Geometry check sheet. Reference: the model listing, model coordinates, mm. Face numbers are marked on the shaded views. A direction names the side the tool comes from. Round coordinates to 2 decimals unless told otherwise and drop trailing zeros. Write each loop counter-clockwise with the first axis right and the second up, starting at its lowest first coordinate (ties: lowest second). Pieces come first, ordered by that corner, then holes.
Item 1: Access from +Z, -Z, +X, -X, +Y, -Y to the whole of each face (thin tool, end or side, straight path). Record for the marked faces 4 and 5.
Item 2: Cross-section at A-A (y = 26.5). Enter the section's corners in (x, z) (1 decimal), then the cut area to 3 significant figures.
Item 3: Cross-section at C-C (x = -82.5). Enter the section's corners in (y, z) (3 decimals).
Item 4: Cross-section at B-B (z = -65.5). Enter the section's corners in (x, y) (3 decimals).
Item 5: Depth check by flat-ended pin: P1, Ø2.5, axis at x = -38.3, y = 51.5, coming from the +Z side; P2, Ø6, axis at x = -35, y = 73.5, coming from the +Z side; P3, Ø2.5, axis at x = -68.9, z = -42.95, coming from the +Y side (3 decimals). Enter the tip coordinate at first touch or a pass-through.
Item 6: Scan lines: probe 1 along Z at (x, y) = (-32.7, 95.5); probe 2 along X at (y, z) = (97, -109.45); probe 3 along Y at (x, z) = (-52.5, -54.5) (3 decimals). Record each from-to range of solid material in increasing order.
Item 7: Draft check along Y on the marked faces 1, 2 and 3. Enter one of: pulls with the +Y half, pulls with the -Y half, needs draft (parallel to the pull), parting line crosses it, or undercut.
Item 8: Cross-section at D-D (y = 44.5). Enter the section's corners in (x, z) (3 decimals), then the cut area to 3 significant figures.
Autodesk Inventor part; units mm, degrees
ref_plane "YZ Plane" through (0, 0, 0) normal (1, 0, 0) x (0, 1, 0)
ref_plane "XZ Plane" through (0, 0, 0) normal (0, 1, 0) x (-1, 0, 0)
ref_plane "XY Plane" through (0, 0, 0) normal (0, 0, 1) x (1, 0, 0)
sketch "Sketch1" plane through (0, 0, 0) normal (1, 0, 0) x (0, 1, 0)
  line L0 (6.35, 0) -> (95.25, 0)
  line L1 (101.6, -6.35) -> (101.6, -146.05)
  line L2 (95.25, -152.4) -> (6.35, -152.4)
  line L3 (0, -146.05) -> (0, -6.35)
  arc A0 (101.6, -6.35) -> (95.25, 0) centre (95.25, -6.35) ccw
  arc A1 (95.25, -152.4) -> (101.6, -146.05) centre (95.25, -146.05) ccw
  arc A2 (0, -146.05) -> (6.35, -152.4) centre (6.35, -146.05) ccw
  arc A3 (6.35, 0) -> (0, -6.35) centre (6.35, -6.35) ccw
  line L4 (92.075, -142.875) -> (92.075, -9.525)
  line L5 (92.075, -9.525) -> (9.525, -9.525)
  line L6 (9.525, -9.525) -> (9.525, -142.875)
  line L7 (9.525, -142.875) -> (92.075, -142.875)
  point P0 (0, 0)
  point P1 (101.6, -152.4)
  point P2 (101.6, 0)
  point P3 (0, -152.4)
  dimension "d0" = 101.6
  dimension "d1" = 152.4
  dimension "d2" = 6.35
  dimension "d3" = 6.35
  dimension "d4" = 9.525
extrude "Extrusion1" add sketch "Sketch1" against normal blind 101.6
sketch "Sketch2" plane through (0, 101.6, -6.35) normal (0, 1, 0) x (1, 0, 0)
  line L0 (0, 0) -> (0, 139.7) construction
  line L1 (0, 69.85) -> (-101.6, 69.85) construction
  line L2 (-101.6, 139.7) -> (-101.6, 0) construction
  line L3 (0, 99.6) -> (-45.4, 99.6) construction
  line L4 (-45.4, 99.6) -> (-45.4, 126.6) construction
  line L5 (-45.4, 126.6) -> (0, 126.6) construction
  line L6 (0, 126.6) -> (0, 99.6) construction
  line L7 (-32.7, 123.1) -> (-12.7, 123.1) construction
  line L8 (-12.7, 123.1) -> (-12.7, 103.1) construction
  line L9 (-12.7, 103.1) -> (-32.7, 103.1) construction
  line L10 (-32.7, 103.1) -> (-32.7, 123.1) construction
  line L11 (-32.7, 123.1) -> (-32.7, 126.6) construction
  line L12 (-32.7, 123.1) -> (-45.4, 123.1) construction
  line L13 (-12.7, 103.1) -> (-12.7, 99.6) construction
  line L14 (-12.7, 103.1) -> (0, 103.1) construction
  circle A0 centre (-32.7, 123.1) radius 1.6
  circle A1 centre (-12.7, 123.1) radius 1.6
  circle A2 centre (-12.7, 103.1) radius 1.6
  circle A3 centre (-32.7, 103.1) radius 1.6
  line L15 (0, 139.7) -> (0, 0) construction
  line L16 (-50.8, 69.85) -> (-50.8, 128.3257) construction
  line L17 (-101.6, 99.6) -> (-56.2, 99.6) construction
  line L18 (-56.2, 99.6) -> (-56.2, 126.6) construction
  line L19 (-56.2, 126.6) -> (-101.6, 126.6) construction
  line L20 (-101.6, 126.6) -> (-101.6, 99.6) construction
  line L21 (-68.9, 123.1) -> (-88.9, 123.1) construction
  line L22 (-88.9, 123.1) -> (-88.9, 103.1) construction
  line L23 (-88.9, 103.1) -> (-68.9, 103.1) construction
  line L24 (-68.9, 103.1) -> (-68.9, 123.1) construction
  line L25 (-68.9, 123.1) -> (-68.9, 126.6) construction
  line L26 (-68.9, 123.1) -> (-56.2, 123.1) construction
  line L27 (-88.9, 103.1) -> (-88.9, 99.6) construction
  line L28 (-88.9, 103.1) -> (-101.6, 103.1) construction
  circle A4 centre (-68.9, 123.1) radius 1.6
  circle A5 centre (-88.9, 123.1) radius 1.6
  circle A6 centre (-88.9, 103.1) radius 1.6
  circle A7 centre (-68.9, 103.1) radius 1.6
  line L29 (0, 40.1) -> (-45.4, 40.1) construction
  line L30 (-45.4, 40.1) -> (-45.4, 13.1) construction
  line L31 (-45.4, 13.1) -> (0, 13.1) construction
  line L32 (0, 13.1) -> (0, 40.1) construction
  line L33 (-32.7, 16.6) -> (-12.7, 16.6) construction
  line L34 (-12.7, 16.6) -> (-12.7, 36.6) construction
  line L35 (-12.7, 36.6) -> (-32.7, 36.6) construction
  line L36 (-32.7, 36.6) -> (-32.7, 16.6) construction
  line L37 (-32.7, 16.6) -> (-32.7, 13.1) construction
  line L38 (-32.7, 16.6) -> (-45.4, 16.6) construction
  line L39 (-12.7, 36.6) -> (-12.7, 40.1) construction
  line L40 (-12.7, 36.6) -> (0, 36.6) construction
  circle A8 centre (-32.7, 16.6) radius 1.6
  circle A9 centre (-12.7, 16.6) radius 1.6
  circle A10 centre (-12.7, 36.6) radius 1.6
  circle A11 centre (-32.7, 36.6) radius 1.6
  line L41 (-68.9, 16.6) -> (-88.9, 16.6) construction
  line L42 (-88.9, 36.6) -> (-68.9, 36.6) construction
  line L43 (-88.9, 36.6) -> (-88.9, 40.1) construction
  line L44 (-88.9, 16.6) -> (-88.9, 36.6) construction
  circle A12 centre (-88.9, 36.6) radius 1.6
  circle A13 centre (-88.9, 16.6) radius 1.6
  line L45 (-101.6, 40.1) -> (-56.2, 40.1) construction
  line L46 (-101.6, 13.1) -> (-101.6, 40.1) construction
  line L47 (-88.9, 36.6) -> (-101.6, 36.6) construction
  line L48 (-56.2, 13.1) -> (-101.6, 13.1) construction
  line L49 (-68.9, 36.6) -> (-68.9, 16.6) construction
  line L50 (-68.9, 16.6) -> (-68.9, 13.1) construction
  circle A14 centre (-68.9, 16.6) radius 1.6
  circle A15 centre (-68.9, 36.6) radius 1.6
  line L51 (-56.2, 40.1) -> (-56.2, 13.1) construction
  line L52 (-68.9, 16.6) -> (-56.2, 16.6) construction
  point P0 (0, -6.35)
  dimension "d7" = 45.4
  dimension "d8" = 27
  dimension "d9" = 20
  dimension "d10" = 20
  dimension "d11" = 3.2
  dimension "d12" = 3.2
  dimension "d13" = 3.2
  dimension "d14" = 3.2
  dimension "d15" = 106.5
extrude "Extrusion2" cut sketch "Sketch2" against normal up to next
sketch "Sketch3" plane through (0, 6.35, -152.4) normal (0, 0, -1) x (-1, 0, 0)
  line L0 (38.3, 45.15) -> (63.3, 45.15) construction
  line L1 (63.3, 45.15) -> (63.3, 20.15) construction
  line L2 (63.3, 20.15) -> (38.3, 20.15) construction
  line L3 (38.3, 20.15) -> (38.3, 45.15) construction
  circle A0 centre (38.3, 45.15) radius 2.1
  circle A1 centre (63.3, 45.15) radius 2.1
  circle A2 centre (63.3, 20.15) radius 2.1
  circle A3 centre (38.3, 20.15) radius 2.1
  line L4 (0, -6.35) -> (101.6, -6.35) construction
  line L5 (38.3, 32.65) -> (0, 32.65) construction
  line L6 (0, 0) -> (0, 88.9) construction
  line L7 (63.3, 32.65) -> (101.6, 32.65) construction
  line L8 (101.6, 88.9) -> (101.6, 0) construction
  dimension "d18" = 25
  dimension "d19" = 25
  dimension "d20" = 4.2
  dimension "d21" = 4.2
  dimension "d22" = 4.2
  dimension "d23" = 4.2
  dimension "d24" = 26.5
extrude "Extrusion3" cut sketch "Sketch3" against normal up to next
sketch "Sketch4" plane through (0, 6.35, 0) normal (0, 0, 1) x (1, 0, 0)
  line L0 (-88.9, 80.5892) -> (-12.7, 80.5892) construction
  line L1 (-12.7, 80.5892) -> (-12.7, 10.7392) construction
  line L2 (-12.7, 10.7392) -> (-88.9, 10.7392) construction
  line L3 (-88.9, 10.7392) -> (-88.9, 80.5892) construction
  line L4 (-88.9, 80.5892) -> (-88.9, 97.6783) construction
  line L5 (-88.9, 80.5892) -> (-101.6, 80.5892) construction
  line L6 (-101.6, 85.725) -> (-101.6, 3.175) construction
  line L7 (-12.7, 10.7392) -> (-12.7, -6.35) construction
  line L8 (0, -6.35) -> (-101.6, -6.35) construction
  line L9 (-12.7, 10.7392) -> (0, 10.7392) construction
  line L10 (0, 85.725) -> (0, 3.175) construction
  circle A0 centre (-12.7, 80.5892) radius 3.175
  circle A1 centre (-12.7, 10.7392) radius 3.175
  circle A2 centre (-88.9, 10.7392) radius 3.175
  circle A3 centre (-88.9, 80.5892) radius 3.175
  circle A4 centre (-63.3, 45.15) radius 2.1
  circle A5 centre (-63.3, 20.15) radius 2.1
  circle A6 centre (-38.3, 45.15) radius 2.1
  circle A7 centre (-38.3, 20.15) radius 2.1
  circle A8 centre (-63.3, 45.15) radius 4.7625
  circle A9 centre (-38.3, 45.15) radius 2.1
  circle A10 centre (-38.3, 45.15) radius 4.7625
  circle A11 centre (-63.3, 20.15) radius 2.1
  circle A12 centre (-63.3, 20.15) radius 4.7625
  circle A13 centre (-38.3, 20.15) radius 2.1
  circle A14 centre (-38.3, 20.15) radius 4.7625
  dimension "d27" = 6.35
  dimension "d28" = 6.35
  dimension "d29" = 6.35
  dimension "d30" = 6.35
  dimension "d31" = 69.85
  dimension "d32" = 76.2
  dimension "d33" = 9.525
  dimension "d34" = 9.525
  dimension "d35" = 9.525
  dimension "d36" = 9.525
extrude "Extrusion4" cut sketch "Sketch4" against normal up to next contours A0 | A1 | A2 | A3 | A4 | A5 | A6 | A7 | A8 | A10 | A12 | A14
thread "Thread1"
thread "Thread2"
thread "Thread3"
thread "Thread4"
sketch "Sketch5" plane through (0, 101.6, -6.35) normal (0, 1, 0) x (1, 0, 0)
  line L0 (21.1594, 98.325) -> (-128.3175, 98.325) construction
  line L1 (0, 146.05) -> (-101.6, 146.05) construction
  circle A0 centre (-32.7, 103.1) radius 1.6 construction
  circle A1 centre (-32.7, 103.1) radius 2.75 construction
  line L2 (0, 3.175) -> (0, 136.525) construction
  line L3 (-101.6, 136.525) -> (-101.6, 3.175) construction
  line L4 (0, 98.325) -> (-101.6, 98.325) construction
  line L5 (-101.6, 98.325) -> (-101.6, 73.325) construction
  line L6 (-101.6, 73.325) -> (0, 73.325) construction
  line L7 (0, 73.325) -> (0, 98.325) construction
  line L8 (-43.3, 78.325) -> (-58.3, 78.325) construction
  line L9 (-58.3, 78.325) -> (-58.3, 93.325) construction
  line L10 (-58.3, 93.325) -> (-43.3, 93.325) construction
  line L11 (-43.3, 93.325) -> (-43.3, 78.325) construction
  line L12 (-43.3, 78.325) -> (0, 78.325) construction
  line L13 (-58.3, 93.325) -> (-101.6, 93.325) construction
  line L14 (-58.3, 93.325) -> (-58.3, 98.325) construction
  line L15 (-43.3, 78.325) -> (-43.3, 73.325) construction
  circle A2 centre (-43.3, 78.325) radius 3.175
  circle A3 centre (-58.3, 78.325) radius 3.175
  circle A4 centre (-58.3, 93.325) radius 3.175
  circle A5 centre (-43.3, 93.325) radius 3.175
  point P0 (0, -6.35)
  dimension "d47" = 47.725
  dimension "d48" = 5.5
  dimension "d49" = 25
  dimension "d50" = 15
  dimension "d51" = 15
  dimension "d52" = 6.35
  dimension "d53" = 6.35
  dimension "d54" = 6.35
  dimension "d55" = 6.35
extrude "Extrusion5" cut sketch "Sketch5" against normal up to next
thread "Thread5"
thread "Thread6"
thread "Thread7"
thread "Thread8"
equation "\"d12\" = d11"
equation "\"d13\" = d11"
equation "\"d14\" = d11"
equation "\"d16\" = d12"
equation "\"d21\" = d20"
equation "\"d22\" = d20"
equation "\"d23\" = d20"
equation "\"d34\" = d33"
equation "\"d35\" = d33"
equation "\"d36\" = d33"
equation "\"d37\" = d33"
equation "\"d53\" = d52"
equation "\"d54\" = d52"
equation "\"d55\" = d52"
properties part number "4in x 6in Steel Rectangular Tubing 4in long Machined"
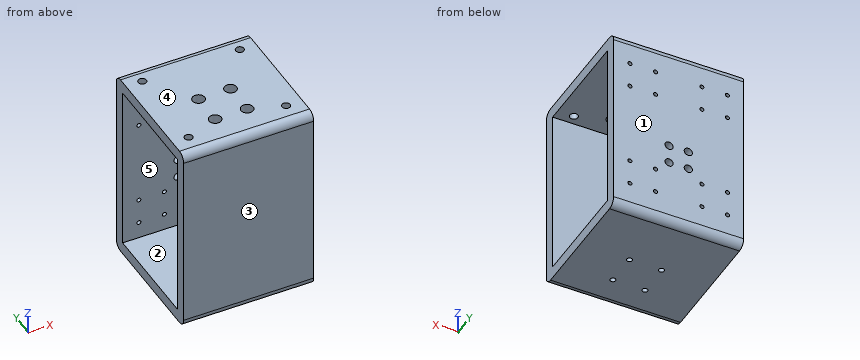
Resolved:
1. face 4: +Z, +X, -X, +Y, -Y
1. face 5: +X, -X
2. outline: (-101.6, -152.4) - (-65.4, -152.4) - (-65.4, -142.9) - (-101.6, -142.9) - close; (-101.6, -9.5) - (-68.1, -9.5) - (-68.1, 0) - (-101.6, 0) - close; (-61.2, -152.4) - (-40.4, -152.4) - (-40.4, -142.9) - (-61.2, -142.9) - close; (-58.5, -9.5) - (-43.1, -9.5) - (-43.1, 0) - (-58.5, 0) - close; (-36.2, -152.4) - (0, -152.4) - (0, -142.9) - (-36.2, -142.9) - close; (-33.5, -9.5) - (0, -9.5) - (0, 0) - (-33.5, 0) - close
2. area: 1,670 mm2
3. outline: (0, -146.05) arc R6.35 ccw to (6.35, -152.4) - (95.25, -152.4) arc R6.35 ccw to (101.6, -146.05) - (101.6, -6.35) arc R6.35 ccw to (95.25, 0) - (6.35, 0) arc R6.35 ccw to (0, -6.35) - close; hole (9.525, -142.875) - (92.075, -142.875) - (92.075, -9.525) - (9.525, -9.525) - close
4. outline: (-101.6, 0) - (0, 0) - (0, 9.525) - (-101.6, 9.525) - close; (-101.6, 92.075) - (0, 92.075) - (0, 101.6) - (-101.6, 101.6) - close
5. P1: passes through
5. P2: stops at z = 0
5. P3: stops at y = 9.525
6. probe 1: z = -152.4 to -131.05, -127.85 to -111.05, -107.85 to -44.55, -41.35 to -24.55, -21.35 to 0
6. probe 2: x = -101.6 to -90.5, -87.3 to -70.5, -67.3 to -34.3, -31.1 to -14.3, -11.1 to 0
6. probe 3: y = 0 to 9.525, 92.075 to 101.6
7. face 1: pulls with the +Y half
7. face 2: undercut
7. face 3: pulls with the -Y half
8. outline: (-101.6, -152.4) - (0, -152.4) - (0, -142.875) - (-101.6, -142.875) - close; (-101.6, -9.525) - (0, -9.525) - (0, 0) - (-101.6, 0) - close
8. area: 1,940 mm2
